from build123d import *

# Parameters (mm, degrees)
F1_R     = 3
F2_R     = 15
F4_T     = -1
F5_R     = 2.1801960973
F6_DEPTH = 25


with BuildPart() as f3:
    # F1 (on offset) → F3 section 0
    with BuildSketch(Plane.XY.offset(60)):
        Circle(F1_R)
    # F2 (on Top) → F3 section 1
    with BuildSketch(Plane.XY):
        Circle(F2_R)
    loft()

    # F4
    f4_openings = [f3.faces().sort_by_distance(p)[0] for p in [
        (0, 0, 0),
    ]]
    offset(amount=F4_T, openings=f4_openings, kind=Kind.INTERSECTION)

    # F5 (on face) → F6 (cut)
    with BuildSketch(Plane(origin=(0, 0, 59), x_dir=(1, 0, 0), z_dir=(0, 0, -1))):
        Circle(F5_R)
    extrude(amount=-F6_DEPTH, mode=Mode.SUBTRACT)


solid = f3.part
Source: CAD feature listing. Evaluate the final solid. Frame: model axes, mm. Round coordinates to 2 decimals unless told otherwise and drop trailing zeros. Loops run counter-clockwise (first coordinate to the right, second up) from the corner with the lowest first, then second, coordinate; pieces in that order, holes last. Notation, with made-up numbers: (13.25, 81.25) -> (48.25, 81.25) arc R30 ccw to (48.25, 106.25) -> close; hole circle Ø1 at (45, -16). An arc over 180 degrees is marked (long way). Answer as a JSON object with one key per item and string values. Group by question number.
Q1. Section query B-B (z = 33.5). Output: boundary loops of the cut face in (x, y), plus the area to 3 significant figures.
Q2. Mould query, pull axis X, two halves, no side actions, for faces 1 (the flat face through (10, -10, 0)), 2 (the cylindrical face through (-2.178, -0.096, 59.493)), 3 (the conical face through (-1.2, 9, 29.6)). Classes: pulls with the +X half, pulls with the -X half, needs draft (parallel to the pull), parting line crosses it, or undercut.
Q3. Ray query, line 1 (X direction, y = 3, z = 16); line 2 (X direction, y = 0, z = 59.45); line 3 (Y direction, x = 0, z = 59.4). Return the intervals inside material, ascending. Write a range as from..to.
Q4. Section query C-C (z = 50.5). Output: boundary loops of the cut face in (x, y).
Q5. Contact query for flat-ended pins moving along their axis: P1, Ø6, axis at x = 6.5, z = 34, coming from the +Y side; P2, Ø1.5, axis at y = 7.5, z = 17.5, coming from the -X side; P3, Ø1, axis at x = 1, z = 33, coming from the +Y side. Output: stop coordinate, or through.
Q6. Section query A-A (x = 0). Output: boundary loops of the cut face in (y, z), plus the area to 3 significant figures.
Completed:
{
 "1": {"outline": "circle Ø16.6 at (0, 0); hole circle Ø14.56 at (0, 0)", "area": "49.9 mm²"},
 "2": {"face 1": "needs draft", "face 2": "undercut", "face 3": "parting line crosses it"},
 "3": {"line 1": "-11.41..-10.35, 10.35..11.41", "line 2": "-3.11..-2.18, 2.18..3.11", "line 3": "-3.12..-2.18, 2.18..3.12"},
 "4": {"outline": "circle Ø9.8 at (0, 0); hole circle Ø7.76 at (0, 0)"},
 "5": {"P1": "y = 7.56", "P2": "x = -9.34", "P3": "y = 8.45"},
 "6": {"outline": "(-15, 0) -> (-13.98, 0) -> (-2.18, 59) -> (-2.18, 60) -> (-3, 60) -> close; (2.18, 59) -> (13.98, 0) -> (15, 0) -> (3, 60) -> (2.18, 60) -> close", "area": "122 mm²"}
}
